from build123d import *

# Parameters (mm, degrees)
BOSS_EXTRUDE1_DEPTH = 11.5
SKETCH2_R           = 3.5
BOSS_EXTRUDE2_DEPTH = 13.5
CUT_EXTRUDE2_DEPTH  = 27.190026728


with BuildPart() as part:
    # Sketch1 → Boss-Extrude1 (new body)
    with BuildSketch(Plane.XY):
        Polygon((5.109549882, -2.95), (5.109549882, 2.95), (0, 5.9), (-5.109549882, 2.95), (-5.109549882, -2.95), (0, -5.9), align=None)
    extrude(amount=BOSS_EXTRUDE1_DEPTH)

    # Sketch2 → Boss-Extrude2 (add)
    with BuildSketch(Plane.XY.offset(11.5)):
        Circle(SKETCH2_R)
    extrude(amount=BOSS_EXTRUDE2_DEPTH)

    # Sketch4 → Cut-Extrude2 (cut, through all)
    with BuildSketch(Plane.XY.offset(25)):
        with BuildLine():
            Line((-0.683282518, 0.925), (0.683282518, 0.925))
            ThreePointArc((0.683282518, 0.925), (1.15, 0), (0.683282518, -0.925))
            Line((0.683282518, -0.925), (-0.683282518, -0.925))
            ThreePointArc((-0.683282518, -0.925), (-1.15, 0), (-0.683282518, 0.925))
        make_face()
    extrude(amount=-CUT_EXTRUDE2_DEPTH, mode=Mode.SUBTRACT)


solid = part.part
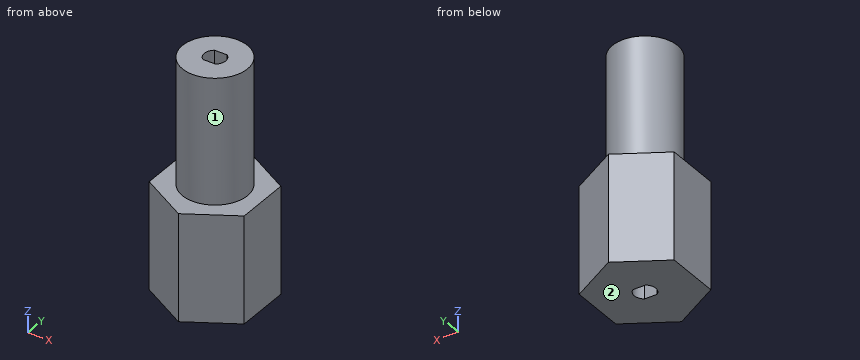
CAD build for the part. Positions are in the model's coordinates, mm. Face numbers are marked on the shaded views. A direction names the side the tool comes from. Coordinates: 2 decimals unless noted, no trailing zeros. Write each loop counter-clockwise with the first axis right and the second up, starting at its lowest first coordinate (ties: lowest second). Pieces come first, ordered by that corner, then holes. Notation, with made-up numbers: M 79,-37 L 91,-37 A9 ccw 91,-28 Z; hole C 38,41 d1. An arc over 180 degrees is marked long. Answer as a JSON object with one key per item and string values. Group by question number.
1) Pin check, flat tips, straight feed: pin 1 Ø1 at (x, z) = (0, 17) entering from +Y; pin 2 Ø6 at (y, z) = (4.5, 13) entering from +X; pin 3 Ø1 at (y, z) = (-3.5, 10.5) entering from +X; pin 4 Ø1 at (x, y) = (4, 1.5) entering from +Z. Stop position of each tip, or through.
2) Wall check: line 1 (Z direction, x = 0.5, y = 4.5); line 2 (X direction, y = 0.75, z = 7.75); line 3 (Y direction, x = 0.25, z = 6.25) (3 decimals). Give the ranges that are in metal, low to high. Write a range as from..to.
3) Saw through at D-D (z = 18). Write the cut outline in (x, y) (3 decimals), plus the area to 3 significant figures.
4) Saw through at C-C (y = -1.25). Write the cut outline in (x, z).
5) Saw through at B-B (z = 5.75). Write the cut outline in (x, y) (3 decimals), plus the area to 3 significant figures.
6) Tool access for the marked faces 1 and 2: list every direction of +Z, -Z, +X, -X, +Y, -Y with a clear straight run to the whole face (end or side of a thin tool).
7) Saw through at A-A (y = 0). Write the cut outline in (x, z).
Values follow:
{
 "1": {"pin 1": "stops at y = 3.5", "pin 2": "stops at x = 5.11", "pin 3": "stops at x = 5.02", "pin 4": "stops at z = 11.5"},
 "2": {"line 1": "z = 0..11.5", "line 2": "x = -5.11..-0.87, 0.87..5.11", "line 3": "y = -5.756..-0.925, 0.925..5.756"},
 "3": {"outline": "C 0,0 d7; hole M -0.683,-0.925 L 0.683,-0.925 A1.15 ccw 0.683,0.925 L -0.683,0.925 A1.15 ccw Z", "area": "34.7 mm2"},
 "4": {"outline": "M -5.11,0 L 5.11,0 L 5.11,11.5 L 3.27,11.5 L 3.27,25 L -3.27,25 L -3.27,11.5 L -5.11,11.5 Z"},
 "5": {"outline": "M -5.11,-2.95 L 0,-5.9 L 5.11,-2.95 L 5.11,2.95 L 0,5.9 L -5.11,2.95 Z; hole M -0.683,-0.925 L 0.683,-0.925 A1.15 ccw 0.683,0.925 L -0.683,0.925 A1.15 ccw Z", "area": "86.7 mm2"},
 "6": {"face 1": "+Z", "face 2": "-Z, +X, -X, +Y, -Y"},
 "7": {"outline": "M -5.11,0 L -1.15,0 L -1.15,25 L -3.5,25 L -3.5,11.5 L -5.11,11.5 Z; M 1.15,0 L 5.11,0 L 5.11,11.5 L 3.5,11.5 L 3.5,25 L 1.15,25 Z"}
}
